```python
from build123d import *

# Parameters (mm, degrees)
F0_W     = 81.5585851669
F0_H     = 43.3602575213
F1_DEPTH = 25.4
F3_DEPTH = 19.558
F5_DEPTH = 11.176


with BuildPart() as f1:
    # F0 (on Top) → F1 (new body)
    with BuildSketch(Plane.XY):
        with Locations((2.322871238, -4.1295485571)):
            Rectangle(F0_W, F0_H)
    extrude(amount=F1_DEPTH)

    # F2 (on face) → F3 (cut)
    with BuildSketch(Plane.XY.offset(25.4)):
        Polygon((-24.2610964924, -4.1295485571), (-38.4564213455, 17.5505802035), (-38.4564213455, -25.8096773177), align=None)
        Polygon((43.1021638215, -25.8096773177), (43.1021638215, 17.5505802035), (28.906840831, -4.1295485571), align=None)
    extrude(amount=-F3_DEPTH, mode=Mode.SUBTRACT)

    # F4 (on face) → F5 (cut)
    with BuildSketch(Plane.XY.offset(25.4)):
        Polygon((-24.2610964924, -4.1295485571), (-38.4564213455, -25.8096773177), (43.1021638215, -25.8096773177), (28.906840831, -4.1295485571), align=None)
    extrude(amount=-F5_DEPTH, mode=Mode.SUBTRACT)


solid = f1.part
```
Read the model definition and answer for the solid it produces. Units are mm, in the model's axes. A direction names the side the tool comes from. Coordinates: 2 decimals unless noted, no trailing zeros. Loops run counter-clockwise (first coordinate to the right, second up) from the corner with the lowest first, then second, coordinate; pieces in that order, holes last. Notation, with made-up numbers: (-20, -36.75) -> (30, -36.75) arc R19 ccw to (30, -15.75) -> close; hole circle Ø3 at (4.25, 8). An arc over 180 degrees is marked (long way). Return JSON: item names as keys, results as strings.
Item 1: Find the intervals of material crossed by probe 1 along Y at (x, z) = (-1, 19.75); probe 2 along Z at (x, y) = (-31, -21.5); probe 3 along Y at (x, z) = (-35, 8.5), in increasing order.
Answers:
{"probe 1": "y = -4.13 to 17.55", "probe 2": "z = 0 to 14.22", "probe 3": "y = -25.81 to -20.53, 12.27 to 17.55"}
Item 2: Find section B-B (y = -23). Determine the outline of the cut face in (x, z), plus the area to 3 significant figures.
Answers:
{"outline": "(-38.46, 0) -> (43.1, 0) -> (43.1, 5.84) -> (41.26, 5.84) -> (41.26, 14.22) -> (-36.62, 14.22) -> (-36.62, 5.84) -> (-38.46, 5.84) -> close", "area": "1,130 mm2"}
Item 3: Flat-ended cylindrical pins translate along their axes: P1, Ø11.5, axis at x = 38.5, y = -8, coming from the +Z side; P2, Ø10, axis at y = 8.5, z = 14.5, coming from the -X side; P3, Ø1, axis at y = 13, z = 15.5, coming from the +X side. Find the tip coordinate at first contact, or state that the pin passes through.
Answers:
{"P1": "stops at z = 5.84", "P2": "stops at x = -35.8", "P3": "stops at x = 40.45"}
Item 4: For a pull along Y with two mould halves and no side action, classify faces 6 (the flat face through (-31.458, -15.121, 10.092)), 7 (the flat face through (2, -4, 0)), 8 (the flat face through (2, 17.551, 13)) as +Y half, -Y half, draft (parallel to the pull), parting line (faces both ways), or undercut.
Answers:
{"face 6": "undercut", "face 7": "draft", "face 8": "+Y half"}
Item 5: For faces 1 (the flat face through (2, -25.81, 7)), 2 (the flat face through (43.102, -4, 3)), 3 (the flat face through (2, -15, 14.224)), 4 (the flat face through (35.905, -14.818, 10.092)), 5 (the flat face through (-33, -4, 5.842)), determine the directions among +Z, -Z, +X, -X, +Y, -Y from which every point of the face is accessible in a straight line to the end or side of a thin tool.
Answers:
{"face 1": "+Z, -Z, +X, -X, -Y", "face 2": "+Z, -Z, +X, +Y, -Y", "face 3": "+Z, +X, -X, -Y", "face 4": "+Z, +X", "face 5": "+Z, -X"}
Item 6: Find section C-C (z = 9.25). Determine the outline of the cut face in (x, y).
Answers:
{"outline": "(-38.46, -25.81) -> (43.1, -25.81) -> (28.91, -4.13) -> (43.1, 17.55) -> (-38.46, 17.55) -> (-24.26, -4.13) -> close"}
Item 7: Find section D-D (x = -31). Determine the outline of the cut face in (y, z).
Answers:
{"outline": "(-25.81, 0) -> (17.55, 0) -> (17.55, 25.4) -> (6.16, 25.4) -> (6.16, 5.84) -> (-14.42, 5.84) -> (-14.42, 14.22) -> (-25.81, 14.22) -> close"}
Item 8: Find section A-A (x = 6.5). Determine the outline of the cut face in (y, z), plus the area to 3 significant figures.
Answers:
{"outline": "(-25.81, 0) -> (17.55, 0) -> (17.55, 25.4) -> (-4.13, 25.4) -> (-4.13, 14.22) -> (-25.81, 14.22) -> close", "area": "859 mm2"}
